Autodesk Inventor part; units mm, degrees
ref_plane "YZ Plane" through (0, 0, 0) normal (1, 0, 0) x (0, 1, 0)
ref_plane "XZ Plane" through (0, 0, 0) normal (0, 1, 0) x (-1, 0, 0)
ref_plane "XY Plane" through (0, 0, 0) normal (0, 0, 1) x (1, 0, 0)
sketch "スケッチ1" plane through (0, 0, 0) normal (0, 0, 1) x (1, 0, 0)
  circle A0 centre (0, 0) radius 4
  circle A1 centre (0, 0) radius 2
  dimension "d0" = 8
  dimension "d1" = 4
extrude "押し出し1" add sketch "スケッチ1" along normal blind 35 contours A0 | A1
sketch "スケッチ2" plane through (0, 0, 35) normal (0, 0, 1) x (1, 0, 0)
  circle A0 centre (0, 0) radius 2
  dimension "d4" = 4
extrude "押し出し2" cut sketch "スケッチ2" against normal blind 8
sketch "スケッチ3" plane through (0, 0, 0) normal (0, 0, -1) x (-1, 0, 0)
  circle A0 centre (0, 0) radius 2
  dimension "d7" = 4
extrude "押し出し3" cut sketch "スケッチ3" against normal blind 8
properties part number "スペーサーm4,35" material "アルミニウム 7075"
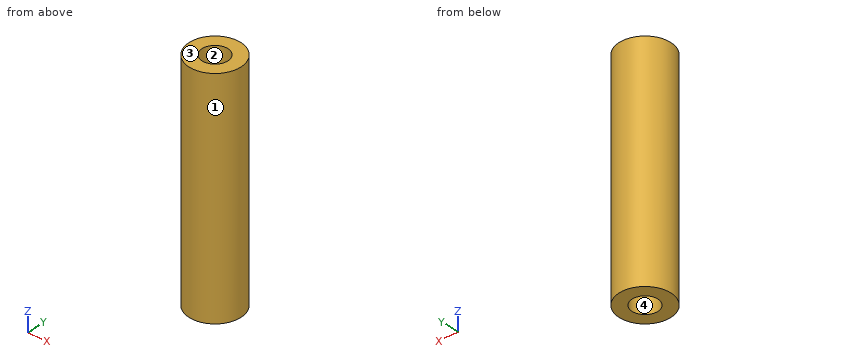
The listing builds one solid part. Answer for the finished solid, in the listing's coordinates (mm). Face numbers are marked on the shaded views. Round coordinates to 2 decimals unless told otherwise and drop trailing zeros. Order: outer loops, then holes, each group sorted by start corner. A loop starts at its lowest first (then second) coordinate and runs counter-clockwise, first axis right, second up. Notation, with made-up numbers: (55.5, 35) -> (100.5, 35) arc R21 cw to (100.5, 73) -> close; hole circle Ø3 at (50.25, 42.25). An arc over 180 degrees is marked (long way). Put each result on its own line as item: value.
Q1. Section D-D, the plane z = 12 is taken. Write down the section's boundary in (x, y), and give its area (3 significant figures).
Results list:
outline: circle Ø8 at (0, 0)
area: 50.3 mm^2
Q2. Determine the mould class of the marked faces 1, 2, 3 and 4 for opening direction Y: pulls with the +Y half, pulls with the -Y half, needs draft (parallel to the pull), parting line crosses it, or undercut.
Results list:
face 1: parting line crosses it
face 2: undercut
face 3: needs draft
face 4: undercut
Q3. Section C-C, the plane z = 30.5 is taken. Write down the section's boundary in (x, y), and give its area (3 significant figures).
Results list:
outline: circle Ø8 at (0, 0); hole circle Ø4 at (0, 0)
area: 37.7 mm^2
Q4. Section A-A, the plane x = 0 is taken. Write down the section's boundary in (y, z), and give its area (3 significant figures).
Results list:
outline: (-4, 0) -> (-2, 0) -> (-2, 8) -> (2, 8) -> (2, 0) -> (4, 0) -> (4, 35) -> (2, 35) -> (2, 27) -> (-2, 27) -> (-2, 35) -> (-4, 35) -> close
area: 216 mm^2
Q5. Consider line 1 along Y through (x, z) = (0, 29.75); line 2 along X through (y, z) = (0.5, 4); line 3 along Z through (x, y) = (0, -0.5). Determine where each line is inside the solid, lowest interval first.
Results list:
line 1: -4 to -2, 2 to 4
line 2: -3.97 to -1.94, 1.94 to 3.97
line 3: 8 to 27
Q6. Each of these flat-tipped pins is pushed along its axis until it touches: P1, Ø3.5, axis at x = 0, y = 0, coming from the -Z side; P2, Ø1.5, axis at x = 3, z = 18, coming from the -Y side; P3, Ø1, axis at x = -2, z = 30.5, coming from the +Y side. Where does it stop, or does it pass through?
Results list:
P1: z = 8
P2: y = -3.31
P3: y = 3.71
